CAD build for the part. Positions are in the model's coordinates, mm. Face numbers are marked on the shaded views. A direction names the side the tool comes from. Give positions to 0.01 mm unless a question says otherwise; leave off trailing zeros. Loops run counter-clockwise (first coordinate to the right, second up) from the corner with the lowest first, then second, coordinate; pieces in that order, holes last. Notation, with made-up numbers: M 46.25,18 L 67.25,18 A16 cw 67.25,34 Z; hole C 2,59 d2. An arc over 180 degrees is marked long. One line per question, with ' | ' between items.
```python
from build123d import *

# Parameters (mm, degrees)
SKETCH1_W                = 108
SKETCH1_H                = 25
BOSS_EXTRUDE1_DEPTH      = 4
CUT_EXTRUDE1_REACH       = 6
SKETCH2_R                = 1.5
SKETCH3_R                = 3.5
SKETCH3_R_2              = 1.5
CUT_EXTRUDE3_DEPTH       = 2
CUT_EXTRUDE4_REACH       = 6
SKETCH4_R                = 1.25
SKETCH5_R                = 3.5
CUT_EXTRUDE5_DEPTH       = 1.7
SKETCH6_W                = 112
SKETCH6_H                = 29
SKETCH6_W_2              = 108
SKETCH6_H_2              = 25
BOSS_EXTRUDE2_DEPTH      = 12
BOSS_EXTRUDE2_DEPTH_BACK = 4
CUT_EXTRUDE8_REACH       = 114
SKETCH10_W               = 17
SKETCH10_H               = 6


with BuildPart() as part:
    # Sketch1 → Boss-Extrude1 (new body)
    with BuildSketch(Plane(origin=(0, 0, 0), x_dir=(1, 0, 0), z_dir=(0, 1, 0))):
        with Locations((11.544540658, 6.287491884)):
            Rectangle(SKETCH1_W, SKETCH1_H)
    extrude(amount=BOSS_EXTRUDE1_DEPTH)

    # Sketch2 → Cut-Extrude1 (cut, up to next)
    with BuildSketch(Plane(origin=(0, 4, 0), x_dir=(1, 0, 0), z_dir=(0, 1, 0)), mode=Mode.PRIVATE) as cut_extrude1_sk1:
        with Locations((-13.455459342, 6.287491884)):
            Circle(SKETCH2_R)
    cut_extrude1_tool1 = extrude(cut_extrude1_sk1.sketch, amount=-CUT_EXTRUDE1_REACH, mode=Mode.PRIVATE) & part.part
    add(cut_extrude1_tool1.solids().sort_by_distance((-13.455459, 4, -6.287492))[0], mode=Mode.SUBTRACT)
    # Sketch2 → Cut-Extrude1 (cut, up to next)
    with BuildSketch(Plane(origin=(0, 4, 0), x_dir=(1, 0, 0), z_dir=(0, 1, 0)), mode=Mode.PRIVATE) as cut_extrude1_sk2:
        with Locations((36.544540658, 6.287491884)):
            Circle(SKETCH2_R)
    cut_extrude1_tool2 = extrude(cut_extrude1_sk2.sketch, amount=-CUT_EXTRUDE1_REACH, mode=Mode.PRIVATE) & part.part
    add(cut_extrude1_tool2.solids().sort_by_distance((36.544541, 4, -6.287492))[0], mode=Mode.SUBTRACT)

    # Sketch3 → Cut-Extrude3 (cut)
    with BuildSketch(Plane(origin=(0, 0, 0), x_dir=(-1, 0, 0), z_dir=(0, -1, 0))):
        with Locations((13.455459342, 6.287491884)):
            Circle(SKETCH3_R)
        with Locations((13.455459342, 6.287491884)):
            Circle(SKETCH3_R_2, mode=Mode.SUBTRACT)
        with Locations((-36.544540658, 6.287491884)):
            Circle(SKETCH3_R)
    extrude(amount=-CUT_EXTRUDE3_DEPTH, mode=Mode.SUBTRACT)

    # Sketch4 → Cut-Extrude4 (cut, up to next)
    with BuildSketch(Plane(origin=(0, 4, 0), x_dir=(1, 0, 0), z_dir=(0, 1, 0)), mode=Mode.PRIVATE) as cut_extrude4_sk1:
        with Locations((21.544540658, 3.787491884)):
            Circle(SKETCH4_R)
    cut_extrude4_tool1 = extrude(cut_extrude4_sk1.sketch, amount=-CUT_EXTRUDE4_REACH, mode=Mode.PRIVATE) & part.part
    add(cut_extrude4_tool1.solids().sort_by_distance((21.544541, 4, -3.787492))[0], mode=Mode.SUBTRACT)
    # Sketch4 → Cut-Extrude4 (cut, up to next)
    with BuildSketch(Plane(origin=(0, 4, 0), x_dir=(1, 0, 0), z_dir=(0, 1, 0)), mode=Mode.PRIVATE) as cut_extrude4_sk2:
        with Locations((1.544540658, 3.787491884)):
            Circle(SKETCH4_R)
    cut_extrude4_tool2 = extrude(cut_extrude4_sk2.sketch, amount=-CUT_EXTRUDE4_REACH, mode=Mode.PRIVATE) & part.part
    add(cut_extrude4_tool2.solids().sort_by_distance((1.544541, 4, -3.787492))[0], mode=Mode.SUBTRACT)

    # Sketch5 → Cut-Extrude5 (cut)
    with BuildSketch(Plane(origin=(0, 4, 0), x_dir=(1, 0, 0), z_dir=(0, 1, 0))):
        with Locations((21.544540658, 3.787491884)):
            Circle(SKETCH5_R)
        with Locations((1.544540658, 3.787491884)):
            Circle(SKETCH5_R)
    extrude(amount=-CUT_EXTRUDE5_DEPTH, mode=Mode.SUBTRACT)

    # Sketch6 → Boss-Extrude2 (add, two sides)
    with BuildSketch(Plane(origin=(0, 4, 0), x_dir=(1, 0, 0), z_dir=(0, 1, 0))) as boss_extrude2_sk:
        with Locations((11.544540658, 6.287491884)):
            Rectangle(SKETCH6_W, SKETCH6_H)
        with Locations((11.544540658, 6.287491884)):
            Rectangle(SKETCH6_W_2, SKETCH6_H_2, mode=Mode.SUBTRACT)
    extrude(amount=BOSS_EXTRUDE2_DEPTH)
    extrude(boss_extrude2_sk.sketch, amount=-BOSS_EXTRUDE2_DEPTH_BACK)

    # Sketch10 → Cut-Extrude8 (cut, up to next)
    with BuildSketch(Plane(origin=(67.544540658, 0, 0), x_dir=(0, 0, -1), z_dir=(1, 0, 0)), mode=Mode.PRIVATE) as cut_extrude8_sk1:
        with Locations((6.287491884, 12)):
            Rectangle(SKETCH10_W, SKETCH10_H)
    cut_extrude8_tool1 = extrude(cut_extrude8_sk1.sketch, amount=-CUT_EXTRUDE8_REACH, mode=Mode.PRIVATE) & part.part
    add(cut_extrude8_tool1.solids().sort_by_distance((67.544541, 12, -6.287492))[0], mode=Mode.SUBTRACT)


solid = part.part
```
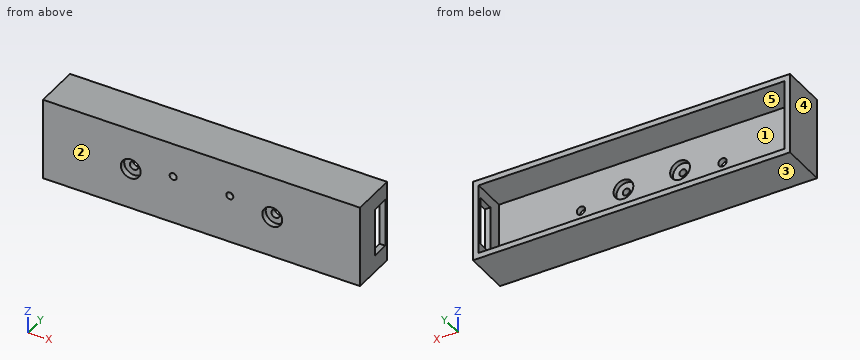
Item 1: Mould opens along Z. For the marked faces 1, 2 and 3 say: pulls with the +Z half, pulls with the -Z half, needs draft (parallel to the pull), parting line crosses it, or undercut.
Conclusion:
face 1: undercut | face 2: needs draft | face 3: pulls with the -Z half
Item 2: Drill centre lines: line 1 along Z through (x, y) = (22.5, 13); line 2 along X through (y, z) = (5, -10); line 3 along X through (y, z) = (3.25, -3). Where is each one in solid material? Low to high. Write a range as [from, to].
Conclusion:
line 1: [-20.79, -18.79], [6.21, 8.21] | line 2: [-44.46, -42.46], [65.54, 67.54] | line 3: [-44.46, -1.87], [4.95, 18.13], [24.95, 67.54]
Item 3: Saw through at C-C on y = 10. Give the cut face in (x, z), and give its area (3 significant figures).
Conclusion:
outline: M -44.46,-20.79 L 67.54,-20.79 L 67.54,-14.79 L 65.54,-14.79 L 65.54,-18.79 L -42.46,-18.79 L -42.46,6.21 L 65.54,6.21 L 65.54,2.21 L 67.54,2.21 L 67.54,8.21 L -44.46,8.21 Z | area: 514 mm²
Item 4: Saw through at A-A on x = 21.5. Give the cut face in (y, z).
Conclusion:
outline: M 0,-20.79 L 16,-20.79 L 16,-18.79 L 4,-18.79 L 4,-7.29 L 2.3,-7.29 L 2.3,-5.04 L 0,-5.04 Z; M 0,-2.54 L 2.3,-2.54 L 2.3,-0.29 L 4,-0.29 L 4,6.21 L 16,6.21 L 16,8.21 L 0,8.21 Z
Item 5: Saw through at B-B on y = 5.75. Give the cut face in (x, z), and give its area (3 significant figures).
Conclusion:
outline: M -44.46,-20.79 L 67.54,-20.79 L 67.54,8.21 L -44.46,8.21 Z; hole M -42.46,-18.79 L 65.54,-18.79 L 65.54,6.21 L -42.46,6.21 Z | area: 548 mm²
Item 6: Drop flat-ended pins along their axis: P1, Ø5.5, axis at x = 1.54, z = -3.79, coming from the +Y side; P2, Ø10, axis at x = 18.5, z = -7, coming from the +Y side; P3, Ø6.5, axis at x = -13.46, z = -6.29, coming from the -Y side. Give the stop position or say it passes through.
Conclusion:
P1: y = 2.3 | P2: y = 4 | P3: y = 2
Item 7: 3-axis set-ups, long thin cutter, end or side, ignore diameter. For the marked faces 4 and 5: which of +Z, -Z, +X, -X, +Y, -Y reach the whole face in a straight line?
Conclusion:
face 4: +Z, -Z, -X, +Y, -Y | face 5: +Y
